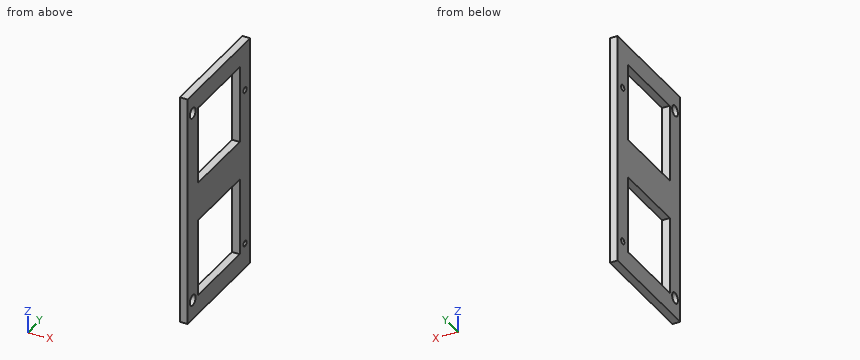
```python
from build123d import *

# Parameters (mm, degrees)
CYLINDER002_R           = 1.5
CYLINDER002_DEPTH       = 4
CYLINDER002_PITCH_ANGLE = 90
CYLINDER003_R           = 1.5
CYLINDER003_DEPTH       = 4
CYLINDER003_PITCH_ANGLE = 90
CYLINDER_R              = 2.75
CYLINDER_DEPTH          = 4
CYLINDER_PITCH_ANGLE    = 90
CYLINDER001_R           = 2.75
CYLINDER001_DEPTH       = 4
CYLINDER001_PITCH_ANGLE = 90
BOX002_W                = 4
BOX002_H                = 40
BOX002_DEPTH            = 40
BOX001_W                = 4
BOX001_H                = 40
BOX001_DEPTH            = 40
BOX_W                   = 4
BOX_H                   = 60
BOX_DEPTH               = 120


with BuildPart() as cilindro002:
    # Cylinder002 → Cylinder002 (new body)
    with BuildSketch(Plane.XY):
        Circle(CYLINDER002_R)
    extrude(amount=CYLINDER002_DEPTH)


with BuildPart() as cilindro002_1:
    # Cylinder002 pitch: moved
    add(cilindro002.part.rotate(Axis((0, 0, 0), (0, 1, 0)), CYLINDER002_PITCH_ANGLE))


with BuildPart() as cilindro002_2:
    # Cylinder002 placement: moved
    add(cilindro002_1.part.moved(Location((0, 55, 95))))


with BuildPart() as cilindro003:
    # Cylinder003 → Cylinder003 (new body)
    with BuildSketch(Plane.XY):
        Circle(CYLINDER003_R)
    extrude(amount=CYLINDER003_DEPTH)


with BuildPart() as cilindro003_1:
    # Cylinder003 pitch: moved
    add(cilindro003.part.rotate(Axis((0, 0, 0), (0, 1, 0)), CYLINDER003_PITCH_ANGLE))


with BuildPart() as cilindro003_2:
    # Cylinder003 placement: moved
    add(cilindro003_1.part.moved(Location((0, 55, 13))))


with BuildPart() as cilindro:
    # Cylinder → Cylinder (new body)
    with BuildSketch(Plane.XY):
        Circle(CYLINDER_R)
    extrude(amount=CYLINDER_DEPTH)


with BuildPart() as cilindro_1:
    # Cylinder pitch: moved
    add(cilindro.part.rotate(Axis((0, 0, 0), (0, 1, 0)), CYLINDER_PITCH_ANGLE))


with BuildPart() as cilindro_2:
    # Cylinder placement: moved
    add(cilindro_1.part.moved(Location((0, 5, 10))))


with BuildPart() as cilindro001:
    # Cylinder001 → Cylinder001 (new body)
    with BuildSketch(Plane.XY):
        Circle(CYLINDER001_R)
    extrude(amount=CYLINDER001_DEPTH)


with BuildPart() as cilindro001_1:
    # Cylinder001 pitch: moved
    add(cilindro001.part.rotate(Axis((0, 0, 0), (0, 1, 0)), CYLINDER001_PITCH_ANGLE))


with BuildPart() as cilindro001_2:
    # Cylinder001 placement: moved
    add(cilindro001_1.part.moved(Location((0, 5, 110))))


with BuildPart() as cubo002:
    # Box002 → Box002 (new body)
    with BuildSketch(Plane(origin=(0, 10, 70), x_dir=(1, 0, 0), z_dir=(0, 0, 1))):
        with Locations((2, 20)):
            Rectangle(BOX002_W, BOX002_H)
    extrude(amount=BOX002_DEPTH)


with BuildPart() as fusion001:
    # Box001 → Box001 (new body)
    with BuildSketch(Plane(origin=(0, 10, 10), x_dir=(1, 0, 0), z_dir=(0, 0, 1))):
        with Locations((2, 20)):
            Rectangle(BOX001_W, BOX001_H)
    extrude(amount=BOX001_DEPTH)

    # Fusion: union Cubo002
    add(cubo002.part)

    # Fusion001: union Cilindro002, Cilindro003, Cilindro, Cilindro001
    add(cilindro002_2.part)
    add(cilindro003_2.part)
    add(cilindro_2.part)
    add(cilindro001_2.part)


with BuildPart() as cut:
    # Box → Box (new body)
    with BuildSketch(Plane.XY):
        with Locations((2, 30)):
            Rectangle(BOX_W, BOX_H)
    extrude(amount=BOX_DEPTH)

    # Cut: cut Fusion001
    add(fusion001.part, mode=Mode.SUBTRACT)


solid = cut.part
```
Source: CAD feature listing. Evaluate the final solid. Frame: model axes, mm. Round coordinates to 2 decimals unless told otherwise and drop trailing zeros. Order: outer loops, then holes, each group sorted by start corner. A loop starts at its lowest first (then second) coordinate and runs counter-clockwise, first axis right, second up. Notation, with made-up numbers: (20.25, 83.5) -> (39.25, 83.5) arc R30 ccw to (39.25, 106.5) -> close; hole circle Ø6 at (37, -7). An arc over 180 degrees is marked (long way). One line per item, written item: value. Start each with the question number.
Q1. Section query B-B (x = 2.7). Return the cut outline in (y, z), plus the area to 3 significant figures.
Q2. Material intervals for probe 1 along Y at (x, z) = (1.1, 95); probe 2 along Z at (x, y) = (0.65, 33); probe 3 along Y at (x, z) = (3.75, 17.5), sorted ascending.
Q3. Section query C-C (z = 95). Return the cut outline in (x, y), plus the area to 3 significant figures.
Q4. Section query A-A (y = 55). Return the cut outline in (x, z).
Findings below:
1. outline: (0, 0) -> (60, 0) -> (60, 120) -> (0, 120) -> close; hole circle Ø5.5 at (5, 10); hole circle Ø5.5 at (5, 110); hole (10, 10) -> (50, 10) -> (50, 50) -> (10, 50) -> close; hole (10, 70) -> (50, 70) -> (50, 110) -> (10, 110) -> close; hole circle Ø3 at (55, 13); hole circle Ø3 at (55, 95)
1. area: 3,940 mm²
2. probe 1: 0 to 10, 50 to 53.5, 56.5 to 60
2. probe 2: 0 to 10, 50 to 70, 110 to 120
2. probe 3: 0 to 10, 50 to 60
3. outline: (0, 0) -> (4, 0) -> (4, 10) -> (0, 10) -> close; (0, 50) -> (4, 50) -> (4, 53.5) -> (0, 53.5) -> close; (0, 56.5) -> (4, 56.5) -> (4, 60) -> (0, 60) -> close
3. area: 68.0 mm²
4. outline: (0, 0) -> (4, 0) -> (4, 11.5) -> (0, 11.5) -> close; (0, 14.5) -> (4, 14.5) -> (4, 93.5) -> (0, 93.5) -> close; (0, 96.5) -> (4, 96.5) -> (4, 120) -> (0, 120) -> close
